Work out the finished part from the listing and answer in its coordinate system (mm). A direction names the side the tool comes from. Coordinates: 2 decimals unless noted, no trailing zeros. Order: outer loops, then holes, each group sorted by start corner. A loop starts at its lowest first (then second) coordinate and runs counter-clockwise, first axis right, second up.
1. Find the intervals of material crossed by probe 1 along Z at (x, y) = (0, -7.5); probe 2 along Z at (x, y) = (0, -48); probe 3 along Y at (x, z) = (-32.5, 9.5), in increasing order.
2. Flat-ended cylindrical pins translate along their axes: pin 1 Ø5 at (x, y) = (4, -26) entering from +Z; pin 2 Ø10 at (y, z) = (-13, -34) entering from -X; pin 3 Ø2 at (x, y) = (-10.5, -24.5) entering from +Z. Find the tip coordinate at first contact, or state that the pin passes through.
3. A tool of negligible diameter and unlimited length cuts with its end or side. For faces 5 (the cylindrical face through (-13.77, -9.39, -61.99)), 6 (the flat face through (-29.1, -19.05, -13.2)), from which of +Z, -Z, +X, -X, +Y, -Y can it reach the whole face along a straight path? Write none if from no direction.
4. The part is cut by section D-D, the plane x = -17. Give the vertices of the cut face in (y, z).
5. The part is cut by section A-A, the plane x = 0. Give the vertices of the cut face in (y, z).
6. The part is cut by section C-C, the plane y = -30.5. Give the vertices of the cut face in (x, z).
7. Determine the mould class of faces 1 (the cylindrical face through (-6.883, -44.806, -30.995)), 2 (the cylindrical face through (-0.827, -9.658, 50.746)), 3 (the flat face through (14, -69.85, -14)), 4 (the cylindrical face through (-15.12, -35.41, -11.59)) for opening direction Z: +Z half, -Z half, draft (parallel to the pull), parting line (faces both ways), or undercut.
8. The part is cut by section B-B, the plane z = 0. Give the vertices of the cut face in (x, y).
```python
from build123d import *

# Parameters (mm, degrees)
F0_R     = 63.5
F1_DEPTH = 19.05
F3_R     = 31.75
F4_DEPTH = 50.8
F5_R     = 19.05
F6_DEPTH = 69.851
F7_R     = 6.35
F8_DEPTH = 19.051


with BuildPart() as f1:
    # F0 (on Front) → F1 (new body)
    with BuildSketch(Plane.XZ):
        Circle(F0_R)
    extrude(amount=F1_DEPTH)

    # F3 (on offset) → F4 (join, through all)
    with BuildSketch(Plane.XZ.offset(69.85)):
        Circle(F3_R)
    extrude(amount=-F4_DEPTH)

    # F5 (on face) → F6 (cut, through all)
    with BuildSketch(Plane.XZ.offset(69.85)):
        Circle(F5_R)
    extrude(amount=-F6_DEPTH, mode=Mode.SUBTRACT)

    # F7 (on face) → F8 (cut, through all)
    with BuildSketch(Plane.XZ.offset(19.05)):
        with Locations((0, 44.45)):
            Circle(F7_R)
    extrude(amount=-F8_DEPTH, mode=Mode.SUBTRACT)


solid = f1.part
```
Geometry says:
1. probe 1: z = -63.5 to -19.05, 19.05 to 38.1, 50.8 to 63.5
1. probe 2: z = -31.75 to -19.05, 19.05 to 31.75
1. probe 3: y = -19.05 to 0
2. pin 1: stops at z = 31.71
2. pin 2: stops at x = -56.49
2. pin 3: stops at z = 30.3
3. face 5: +Y, -Y
3. face 6: -Y
4. outline: (-69.85, -26.82) - (-19.05, -26.82) - (-19.05, -61.18) - (0, -61.18) - (0, -8.6) - (-69.85, -8.6) - close; (-69.85, 8.6) - (0, 8.6) - (0, 61.18) - (-19.05, 61.18) - (-19.05, 26.82) - (-69.85, 26.82) - close
5. outline: (-69.85, -31.75) - (-19.05, -31.75) - (-19.05, -63.5) - (0, -63.5) - (0, -19.05) - (-69.85, -19.05) - close; (-69.85, 19.05) - (0, 19.05) - (0, 38.1) - (-19.05, 38.1) - (-19.05, 31.75) - (-69.85, 31.75) - close; (-19.05, 50.8) - (0, 50.8) - (0, 63.5) - (-19.05, 63.5) - close
6. outline: circle Ø63.5 at (0, 0); hole circle Ø38.1 at (0, 0)
7. face 1: parting line
7. face 2: undercut
7. face 3: draft
7. face 4: undercut
8. outline: (-63.5, -19.05) - (-31.75, -19.05) - (-31.75, -69.85) - (-19.05, -69.85) - (-19.05, 0) - (-63.5, 0) - close; (19.05, -69.85) - (31.75, -69.85) - (31.75, -19.05) - (63.5, -19.05) - (63.5, 0) - (19.05, 0) - close
